Build history of the part. All positions in model axes, mm. A direction names the side the tool comes from. Coordinates: 2 decimals unless noted, no trailing zeros. Write each loop counter-clockwise with the first axis right and the second up, starting at its lowest first coordinate (ties: lowest second). Pieces come first, ordered by that corner, then holes.
from build123d import *

# Parameters (mm, degrees)
SKETCH1_R            = 17.6
SKETCH1_R_2          = 8.1
BOSS_EXTRUDE1_DEPTH  = 5
CUT_EXTRUDE1_DEPTH   = 2.6
M3_CLEARANCE_HOLE1_D = 3.2
CIRPATTERN1_COUNT    = 6


with BuildPart() as part:
    # Sketch1 → Boss-Extrude1 (new body)
    with BuildSketch(Plane(origin=(0, 0, 0), x_dir=(1, 0, 0), z_dir=(0, 1, 0))):
        with Locations(Location((0, 0, 0), (0, 0, 270))):
            Circle(SKETCH1_R)
        with Locations(Location((0, 0, 0), (0, 0, 270))):
            Circle(SKETCH1_R_2, mode=Mode.SUBTRACT)
    extrude(amount=BOSS_EXTRUDE1_DEPTH)

    # Sketch2 → Cut-Extrude1 (cut)
    with BuildSketch(Plane.XZ):
        Polygon((13.5, 3.233161507), (10.7, 1.616580754), (10.7, -1.616580754), (13.5, -3.233161507), (16.3, -1.616580754), (16.3, 1.616580754), align=None)
    cut_extrude1 = extrude(amount=-CUT_EXTRUDE1_DEPTH, mode=Mode.SUBTRACT)

    # M3 Clearance Hole1 (through all)
    with Locations(Plane(origin=(0, 2.6, 0), x_dir=(-1, 0, 0), z_dir=(0, -1, 0))):
        with Locations((-13.5, 0)):
            m3_clearance_hole1 = Hole(M3_CLEARANCE_HOLE1_D / 2)

    # CirPattern1: Cut-Extrude1, M3 Clearance Hole1 ×6 about axis
    cirpattern1_axis = Axis((0, 0, 0), (0, 1, 0))
    add([cut_extrude1.rotate(cirpattern1_axis, i * 360 / CIRPATTERN1_COUNT) for i in range(1, CIRPATTERN1_COUNT)], mode=Mode.SUBTRACT)
    add([m3_clearance_hole1.rotate(cirpattern1_axis, i * 360 / CIRPATTERN1_COUNT) for i in range(1, CIRPATTERN1_COUNT)], mode=Mode.SUBTRACT)


solid = part.part
(1) Flat gauge pins, fed straight in: P1, Ø1.9, axis at x = -13.5, z = 0, coming from the +Y side; P2, Ø1, axis at x = 14, y = 2, coming from the +Z side; P3, Ø3, axis at y = 2, z = 11, coming from the +X side; P4, Ø4, axis at x = 6.75, z = 11.69, coming from the -Y side. Where does each tip first touch, or does it go through?
(2) 3-axis set-ups, long thin cutter, end or side, ignore diameter. For faces 1 (the cylindrical face through (-7.93, 3.82, 10.61)), 2 (the flat face through (5.33, 1.28, 9.28)): which of +Z, -Z, +X, -X, +Y, -Y reach the whole face in a straight line?
(3) Slice it at D-D, the plane y = 0.95. Give the number of separate pieces and of enclosed holes in the cut face, and give its area (3 significant figures).
(4) Slice it at B-B, the plane x = 4.5. List the corners of the cut face in (y, z) (3 decimals), and give its area (3 significant figures).
(5) Probe L1, parallel to X at y = 2.2, z = -11; L2, parallel to X at y = 0.2, z = 14; L3, parallel to Z at x = 9, y = 0.55. List the from-to ranges inside material, lowest first.
(6) Slice it at C-C, the plane z = -7.5. List the corners of the cut face in (x, y).
(7) Slice it at A-A, the plane z = 0. List the corners of the cut face in (x, y), and give its area (3 significant figures).
Results:
1. P1: passes through
1. P2: stops at z = 11.29
1. P3: stops at x = 14.82
1. P4: stops at y = 2.6
2. face 1: +Y, -Y
2. face 2: -Y
3. separate pieces: 1
3. enclosed holes: 7
3. area: 604 mm2
4. outline: (0, -17.015) - (5, -17.015) - (5, -6.735) - (0, -6.735) - (0, -9.757) - (2.6, -9.757) - (2.6, -13.625) - (0, -13.625) - close; (0, 6.735) - (5, 6.735) - (5, 17.015) - (0, 17.015) - (0, 13.625) - (2.6, 13.625) - (2.6, 9.757) - (0, 9.757) - close
4. area: 82.7 mm2
5. L1: x = -13.74 to -9.55, -3.95 to 3.95, 9.55 to 13.74
5. L2: x = -10.67 to -8.35, -5.15 to 5.15, 8.35 to 10.67
5. L3: z = -15.12 to -13.63, -9.76 to 9.76, 13.63 to 15.12
6. outline: (-15.92, 0) - (-3.06, 0) - (-3.06, 5) - (-15.92, 5) - close; (3.06, 0) - (15.92, 0) - (15.92, 5) - (3.06, 5) - close
7. outline: (-17.6, 0) - (-16.3, 0) - (-16.3, 2.6) - (-15.1, 2.6) - (-15.1, 5) - (-17.6, 5) - close; (-11.9, 2.6) - (-10.7, 2.6) - (-10.7, 0) - (-8.1, 0) - (-8.1, 5) - (-11.9, 5) - close; (8.1, 0) - (10.7, 0) - (10.7, 2.6) - (11.9, 2.6) - (11.9, 5) - (8.1, 5) - close; (15.1, 2.6) - (16.3, 2.6) - (16.3, 0) - (17.6, 0) - (17.6, 5) - (15.1, 5) - close
7. area: 50.5 mm2
